from build123d import *

# Parameters (mm, degrees)
CROQUIS1_W              = 101.54
CROQUIS1_H              = 25.72
CROQUIS1_W_2            = 98.34
CROQUIS1_H_2            = 22.52
SALIENTE_EXTRUIR1_DEPTH = 91.02
CROQUIS2_W              = 98.34
CROQUIS2_H              = 182.04
CORTAR_EXTRUIR1_DEPTH   = 6.04


with BuildPart() as part:
    # Croquis1 → Saliente-Extruir1 (new, symmetric)
    with BuildSketch(Plane.XY):
        with Locations((-27.147074341, -0.246714628)):
            Rectangle(CROQUIS1_W, CROQUIS1_H)
        with Locations((-27.147074341, -0.246714628)):
            Rectangle(CROQUIS1_W_2, CROQUIS1_H_2, mode=Mode.SUBTRACT)
    extrude(amount=SALIENTE_EXTRUIR1_DEPTH, both=True)

    # Croquis2 → Cortar-Extruir1 (cut)
    with BuildSketch(Plane(origin=(0, 12.613285372, 0), x_dir=(1, 0, 0), z_dir=(0, 1, 0))):
        with Locations((-27.147074341, 0)):
            Rectangle(CROQUIS2_W, CROQUIS2_H)
    extrude(amount=-CORTAR_EXTRUIR1_DEPTH, mode=Mode.SUBTRACT)


solid = part.part
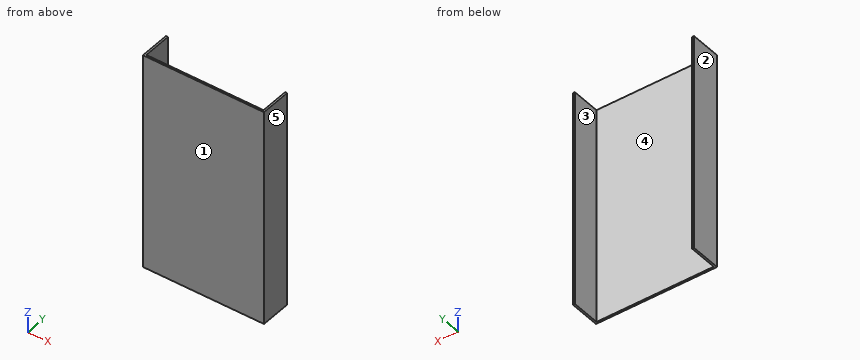
Can you work these out from the model? Positions are in its coordinate system, mm. Face numbers are marked on the shaded views. A direction names the side the tool comes from. Round coordinates to 2 decimals unless told otherwise and drop trailing zeros. Order: outer loops, then holes, each group sorted by start corner. A loop starts at its lowest first (then second) coordinate and runs counter-clockwise, first axis right, second up. Notation, with made-up numbers: (30, -14.75) -> (42, -14.75) arc R10 ccw to (42, -6.75) -> close; hole circle Ø6 at (68.5, 59.25). An arc over 180 degrees is marked (long way). Write each question's results on one line, items separated by ' | '. Start each with the question number.
Item 1: Please list where these lines run through material, in increasing order: L1, parallel to X at y = 8.5, z = 39.5; L2, parallel to Y at x = -13, z = 76.5.
Item 2: If we section it at B-B, the plane z = 54: Write out the boundary of the cut face in (x, y), then the cut area to 3 significant figures.
Item 3: Which directions (+Z, -Z, +X, -X, +Y, -Y) give clear straight access to the entire face, cutting with the end or side of a thin tool? Please do the marked faces 4 and 5.
Item 4: If we section it at C-C, the plane x = 4: Write out the boundary of the cut face in (y, z).
Item 5: Will this pin go through, and if not, where does the flat tip stop? pin 1 (4 mm diameter, centred on x = -19, z = 6, fed in from +Y).
Item 6: Thinking about a two-plate mould opening in X: for the marked faces 1, 2 and 3, which applies, +X half, -X half, draft (parallel to the pull), parting line (faces both ways), or undercut?
Item 7: If we section it at A-A, the plane y = 3.75: Write out the boundary of the cut face in (x, z).
Results:
1) L1: x = -77.92 to -76.32, 22.02 to 23.62 | L2: y = -13.11 to -11.51
2) outline: (-77.92, -13.11) -> (23.62, -13.11) -> (23.62, 12.61) -> (22.02, 12.61) -> (22.02, -11.51) -> (-76.32, -11.51) -> (-76.32, 12.61) -> (-77.92, 12.61) -> close | area: 240 mm2
3) face 4: +Z, -Z, +Y | face 5: +Z, -Z, +X, +Y, -Y
4) outline: (-13.11, -91.02) -> (-11.51, -91.02) -> (-11.51, 91.02) -> (-13.11, 91.02) -> close
5) pin 1: stops at y = -11.51
6) face 1: draft | face 2: -X half | face 3: undercut
7) outline: (-77.92, -91.02) -> (-76.32, -91.02) -> (-76.32, 91.02) -> (-77.92, 91.02) -> close; (22.02, -91.02) -> (23.62, -91.02) -> (23.62, 91.02) -> (22.02, 91.02) -> close
